Work out the finished part from the listing and answer in its coordinate system (mm). Face numbers are marked on the shaded views. A direction names the side the tool comes from. Round coordinates to 2 decimals unless told otherwise and drop trailing zeros. Order: outer loops, then holes, each group sorted by start corner. A loop starts at its lowest first (then second) coordinate and runs counter-clockwise, first axis right, second up. Notation, with made-up numbers: (-14.5, 13.25) - (7.5, 13.25) arc R10 cw to (7.5, 32.25) - close; hole circle Ø8 at (-25.75, -7.5). An arc over 180 degrees is marked (long way). Use one line per item in the form item = value. Start each with the question number.
Q1. The part is cut by section C-C on y = 28.5. Determine the outline of the cut face in (x, z).
Q2. The part is cut by section A-A on z = 0. Determine the outline of the cut face in (x, y).
Q3. The part is cut by section D-D on x = -4.25. Determine the outline of the cut face in (y, z).
Q4. Which of the six approach directions +Z, -Z, +X, -X, +Y, -Y give full straight-line access (tool end or side, diameter ignored) to the marked faces 1 and 2?
Q5. Given P1, Ø10, axis at y = 32.5, z = -12, coming from the -X side; P2, Ø15, axis at x = 6, z = 5, coming from the +Y side, each flat-ended and moving along its own axis, determine where each tip first touches the part or whether it passes through.
Q6. The part is cut by section B-B on x = 0. Determine the outline of the cut face in (y, z).
Q7. Find the intervals of material crossed by line 1 (Y direction, x = 11.5, z = 4.25); line 2 (Z direction, x = -2.25, y = 55), in increasing order. Write a range as [from, to].
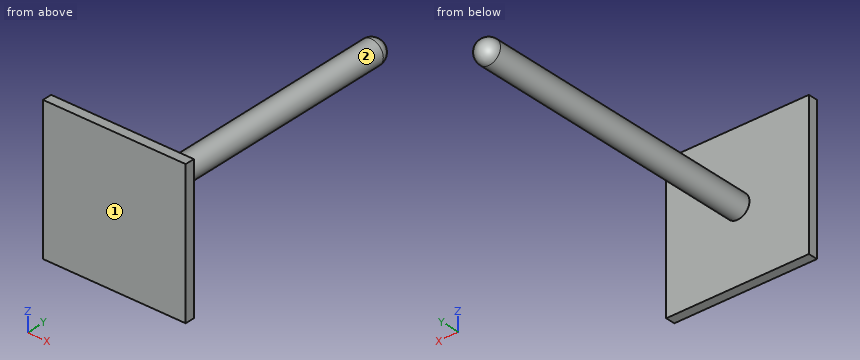
Autodesk Inventor part; units mm, degrees
ref_plane "YZ Plane" through (0, 0, 0) normal (1, 0, 0) x (0, 1, 0)
ref_plane "XZ Plane" through (0, 0, 0) normal (0, 1, 0) x (-1, 0, 0)
ref_plane "XY Plane" through (0, 0, 0) normal (0, 0, 1) x (1, 0, 0)
sketch "Sketch1" plane through (0, 0, 0) normal (0, 1, 0) x (-1, 0, 0)
  line L0 (15, 15) -> (-15, 15)
  line L1 (-15, 15) -> (-15, -15)
  line L2 (-15, -15) -> (15, -15)
  line L3 (15, -15) -> (15, 15)
  point P0 (0, 0)
  point P1 (15, 0)
  point P2 (0, 15)
  dimension "d0" = 30
  dimension "d1" = 30
  dimension "d2" = 0
  dimension "d3" = 0
extrude "Extrusion1" add sketch "Sketch1" along normal blind 2
sketch "Sketch2" plane through (0, 2, 0) normal (0, 1, 0) x (1, 0, 0)
  circle A0 centre (0, 0) radius 2.5
  dimension "d6" = 5
extrude "Extrusion2" add sketch "Sketch2" along normal blind 61.394
sketch "Sketch3" plane through (0, 63.394, 0) normal (0, 1, 0) x (1, 0, 0)
  point P0 (0, 0)
sketch "Sketch4" plane through (0, 0, 0) normal (1, 0, 0) x (0, 1, 0)
  line L0 (63.394, -2.5) -> (63.394, 2.5)
  circle A0 centre (63.394, 0) radius 2.5
  line L1 (65.894, 0) -> (63.394, 0)
  line L2 (63.394, 0) -> (63.394, -2.5)
  line L3 (65.894, 0) -> (66.7994, 0)
  point P0 (0, 0)
  dimension "d6" = 5
  dimension "d9" = 5
revolve "Revolution3" add sketch "Sketch4" angle 360 about axis through (0, 65.894, 0) along (0, -1, 0) picked at (64.2751, -1.4023) contours L0 L1 A0
properties part number "Pivot"
Found:
q1.outline = circle Ø5 at (0, 0)
q2.outline = (-15, 0) - (15, 0) - (15, 2) - (2.5, 2) - (2.5, 63.39) arc R2.5 ccw to (-2.5, 63.39) - (-2.5, 2) - (-15, 2) - close
q3.outline = (0, -15) - (2, -15) - (2, 15) - (0, 15) - close
q4.face_1 = +Z, -Z, +X, -X, -Y
q4.face_2 = +Y
q5.P1 = through
q5.P2 = 65.87
q6.outline = (0, -15) - (2, -15) - (2, -2.5) - (63.39, -2.5) arc R2.5 ccw to (63.39, 2.5) - (2, 2.5) - (2, 15) - (0, 15) - close
q7.line_1 = [0, 2]
q7.line_2 = [-1.09, 1.09]
